from build123d import *

# Parameters (mm, degrees)
SKETCH1_W                                           = 25.41
SKETCH1_H                                           = 18.5
BOSS_EXTRUDE1_DEPTH                                 = 15
F_2_56_TAPPED_HOLE1_D                               = 1.778
F_2_56_TAPPED_HOLE1_DEPTH                           = 7.46583491
F_2_56_TAPPED_HOLE1_TIP                             = 0.53416509
SKETCH5_R                                           = 3
CUT_EXTRUDE1_DEPTH                                  = 3
CBORE_FOR_2_BINDING_HEAD_MACHINE_SCREW1_D           = 2.4384
CBORE_FOR_2_BINDING_HEAD_MACHINE_SCREW1_CBORE_D     = 5.55752
CBORE_FOR_2_BINDING_HEAD_MACHINE_SCREW1_CBORE_DEPTH = 7.269988


with BuildPart() as part:
    # Sketch1 → Boss-Extrude1 (new body)
    with BuildSketch(Plane(origin=(0, 0, 0), x_dir=(1, 0, 0), z_dir=(0, 1, 0))):
        with Locations((12.705, 9.25)):
            Rectangle(SKETCH1_W, SKETCH1_H)
    extrude(amount=BOSS_EXTRUDE1_DEPTH)

    # #2-56 Tapped Hole1
    with Locations(Plane(origin=(0, 0, 0), x_dir=(-1, 0, 0), z_dir=(0, -1, 0))):
        with Locations((-23.91, 17), (-23.91, 1.5), (-1.5, 1.5), (-1.5, 17)):
            Hole(F_2_56_TAPPED_HOLE1_D / 2, depth=F_2_56_TAPPED_HOLE1_DEPTH)
            with Locations((0, 0, -(F_2_56_TAPPED_HOLE1_DEPTH + F_2_56_TAPPED_HOLE1_TIP / 2))):  # 118° drill point
                Cone(0, F_2_56_TAPPED_HOLE1_D / 2, F_2_56_TAPPED_HOLE1_TIP, mode=Mode.SUBTRACT)

    # Sketch5 → Cut-Extrude1 (cut)
    with BuildSketch(Plane.XZ):
        with Locations((12.705, -9.25)):
            Circle(SKETCH5_R)
    extrude(amount=-CUT_EXTRUDE1_DEPTH, mode=Mode.SUBTRACT)

    # CBORE for #2 Binding Head Machine Screw1 (through all)
    with Locations(Plane(origin=(0, 0, 0), x_dir=(-1, 0, 0), z_dir=(0, -1, 0))):
        with Locations((-23.91, 9.25), (-1.5, 9.25)):
            CounterBoreHole(CBORE_FOR_2_BINDING_HEAD_MACHINE_SCREW1_D / 2, CBORE_FOR_2_BINDING_HEAD_MACHINE_SCREW1_CBORE_D / 2, CBORE_FOR_2_BINDING_HEAD_MACHINE_SCREW1_CBORE_DEPTH)


solid = part.part
For this review, take the finished solid that the model builds, in its own axes (mm). A direction names the side the tool comes from. Give positions to 0.01 mm unless a question says otherwise; leave off trailing zeros. Order: outer loops, then holes, each group sorted by start corner. A loop starts at its lowest first (then second) coordinate and runs counter-clockwise, first axis right, second up. Notation, with made-up numbers: M 57,1.5 L 63,1.5 A11 cw 63,11.5 Z; hole C -16.5,73 d9. An arc over 180 degrees is marked long. Answer in a Markdown table with one row per item. Add a question column.
(1) Wall thickness on probe 1 along X at (y, z) = (6.75, -2); probe 2 along Z at (x, y) = (23.91, 9.75); probe 3 along Y at (x, z) = (23.5, -10.5): over which ranges is each line inside the solid? List them lowest first. Write a range as [from, to].
(2) For faces 4 (the face through (22.94, 11.19, -8.51)), 5 (the face through (23.255, 3.785, -17.601)), list the 3-axis set-ups (+Z, -Z, +X, -X, +Y, -Y) from which the entire face can be reached by the end or side of a thin tool; tool diameter is ignored.
(3) Consider section C-C on y = 1.5. State the section outline as (x, z) points (3 decimals).
(4) For pin 1 (1.6 mm diameter, centred on x = 1.5, z = -1.5, fed in from -Y); pin 2 (1.3 mm diameter, centred on x = 1.5, z = -8, fed in from -Y), all flat-tipped, find the tip position at first contact; note any pin that passes through.
(5) Consider section D-D on x = 11. State the section outline as (y, z) points, and give its area (3 significant figures).
(6) Mouldability with a two-part tool opening along Y and no side actions: class faces 1 (the face through (1.53, 7.91, -1.35)), 2 (the face through (13, 15, -9)), 3 (the face through (13, 7, -18.5)) as +Y half, -Y half, draft (parallel to the pull), parting line (faces both ways), or undercut.
(7) Consider section B-B on y = 9.5. State the section outline as (x, z) points.
(8) Consider section A-A on z = -9.25. State the section outline as (x, y) points (3 decimals), and give its area (3 significant figures).
Evaluation:
| question | item | result |
|---|---|---|
| 1 | probe 1 | x = [0, 0.76], [2.24, 23.17], [24.65, 25.41] |
| 1 | probe 2 | z = [-18.5, -10.47], [-8.03, 0] |
| 1 | probe 3 | y = [7.27, 15] |
| 2 | face 4 | +Y, -Y |
| 2 | face 5 | -Y |
| 3 | outline | M 0,-18.5 L 25.41,-18.5 L 25.41,-11.589 A2.779 cw long 25.41,-6.911 L 25.41,0 L 0,0 L 0,-6.911 A2.779 cw long 0,-11.589 Z; hole C 1.5,-17 d1.778; hole C 1.5,-1.5 d1.778; hole C 12.705,-9.25 d6; hole C 23.91,-17 d1.778; hole C 23.91,-1.5 d1.778 |
| 4 | pin 1 | stops at y = 7.52 |
| 4 | pin 2 | stops at y = 7.27 |
| 5 | outline | M 0,-18.5 L 15,-18.5 L 15,0 L 0,0 L 0,-6.78 L 3,-6.78 L 3,-11.72 L 0,-11.72 Z |
| 5 | area | 263 mm^2 |
| 6 | face 1 | -Y half |
| 6 | face 2 | +Y half |
| 6 | face 3 | draft |
| 7 | outline | M 0,-18.5 L 25.41,-18.5 L 25.41,0 L 0,0 Z; hole C 1.5,-9.25 d2.44; hole C 23.91,-9.25 d2.44 |
| 8 | outline | M 0,7.27 L 0.281,7.27 L 0.281,15 L 0,15 Z; M 2.719,7.27 L 4.279,7.27 L 4.279,0 L 9.705,0 L 9.705,3 L 15.705,3 L 15.705,0 L 21.131,0 L 21.131,7.27 L 22.691,7.27 L 22.691,15 L 2.719,15 Z; M 25.129,7.27 L 25.41,7.27 L 25.41,15 L 25.129,15 Z |
| 8 | area | 263 mm^2 |
